Design review of the part shown in the three views and the two pictorial views. Dimensions are in mm from the part's minimum x, y and z. A direction names the side the tool comes from. Give positions to 0.01 mm unless a question says otherwise; leave off trailing zeros. Loops run counter-clockwise (first coordinate to the right, second up) from the corner with the lowest first, then second, coordinate; pieces in that order, holes last. Notation, with made-up numbers: (76.25, -5) - (131.25, -5) arc R14 ccw to (131.25, 14) - close; hole circle Ø3 at (29.5, 76.25). An arc over 180 degrees is marked (long way). Answer in a Markdown table with one row per item.
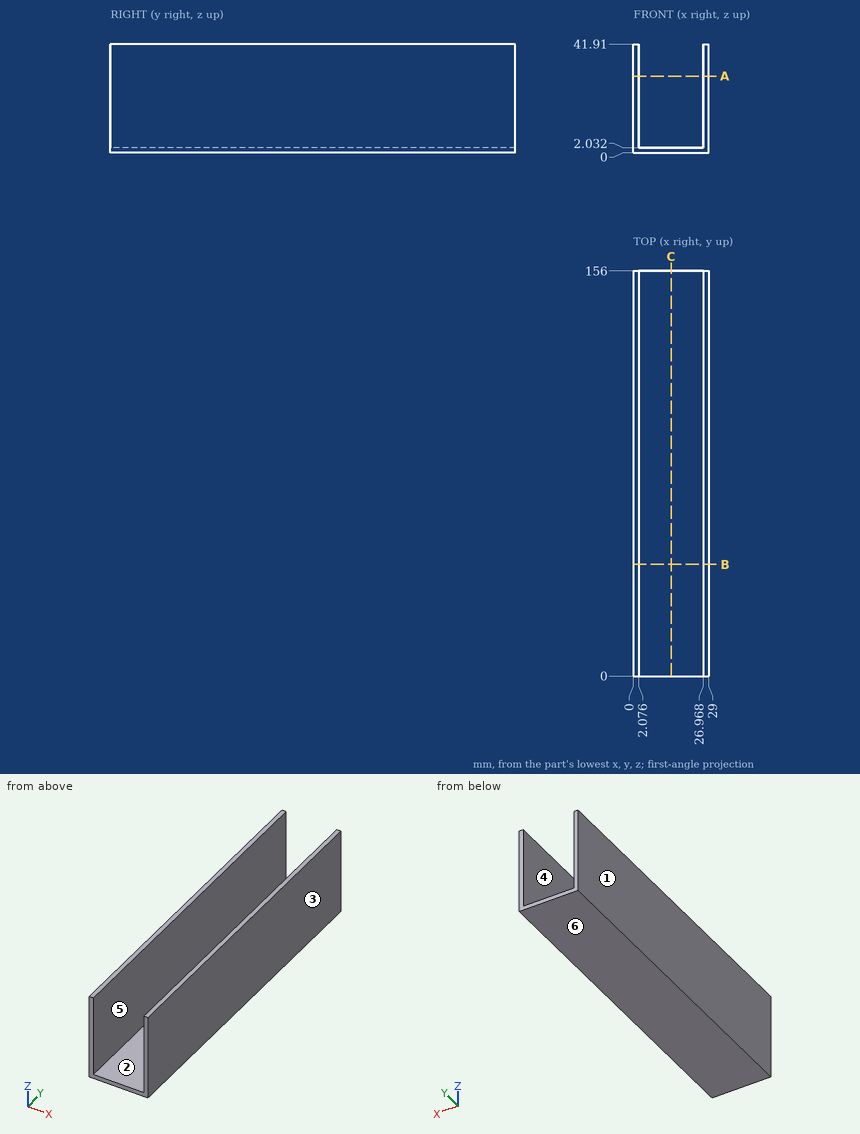
1. We need section C-C, the plane x = 14.5. Give the boundary of the cut face in (y, z).
Values:
| item | result |
|---|---|
| outline | (0, 0) - (156, 0) - (156, 2.03) - (0, 2.03) - close |
2. We need section A-A, the plane z = 29.5. Give the boundary of the cut face in (x, y).
Values:
| item | result |
|---|---|
| outline | (0, 0) - (2.08, 0) - (2.08, 156) - (0, 156) - close; (26.97, 0) - (29, 0) - (29, 156) - (26.97, 156) - close |
3. We need section B-B, the plane y = 43. Give the boundary of the cut face in (x, z).
Values:
| item | result |
|---|---|
| outline | (0, 0) - (29, 0) - (29, 41.91) - (26.97, 41.91) - (26.97, 2.03) - (2.08, 2.03) - (2.08, 41.91) - (0, 41.91) - close |
4. For the marked faces 1 and 2, list the 3-axis set-ups (+Z, -Z, +X, -X, +Y, -Y) from which the entire face can be reached by the end or side of a thin tool; tool diameter is ignored.
Values:
| item | result |
|---|---|
| face 1 | +Z, -Z, -X, +Y, -Y |
| face 2 | +Z, +Y, -Y |
5. Wall thickness on line 1 (X direction, y = 94.5, z = 31.5); line 2 (Z direction, x = 10.5, y = 102): over which ranges is each line inside the solid? List them lowest first. Write a range as [from, to].
Values:
| item | result |
|---|---|
| line 1 | x = [0, 2.08], [26.97, 29] |
| line 2 | z = [0, 2.03] |
6. Clearance check with flat-ended pins moving along their axes: pin 1 (4 mm diameter, centred on x = 26, z = 32, fed in from +Y); pin 2 (3 mm diameter, centred on x = 5.5, z = 30.5, fed in from +Y); pin 3 (12.5 mm diameter, centred on x = 18.5, y = 81, fed in from +Z). State where each tip first meets the part, or that it passes through.
Values:
| item | result |
|---|---|
| pin 1 | stops at y = 156 |
| pin 2 | passes through |
| pin 3 | stops at z = 2.03 |
7. Mouldability with a two-part tool opening along X and no side actions: class the marked faces 3, 4, 5 and 6 as released by +X, released by -X, zero draft, split by the parting line, or undercut.
Values:
| item | result |
|---|---|
| face 3 | released by +X |
| face 4 | undercut |
| face 5 | undercut |
| face 6 | zero draft |
